Autodesk Inventor part; units mm, degrees
ref_plane "YZ Plane" through (0, 0, 0) normal (1, 0, 0) x (0, 1, 0)
ref_plane "XZ Plane" through (0, 0, 0) normal (0, 1, 0) x (-1, 0, 0)
ref_plane "XY Plane" through (0, 0, 0) normal (0, 0, 1) x (1, 0, 0)
sketch "Sketch1" plane through (0, 0, 0) normal (0, 1, 0) x (-1, 0, 0)
  line L0 (0, 0) -> (-12.7, 0)
  line L1 (-12.7, 0) -> (-12.7, -19.05)
  line L2 (-12.7, -19.05) -> (0, -19.05)
  line L3 (0, -19.05) -> (0, 0)
  line L4 (-12.7, -9.525) -> (0, -9.525)
  circle A0 centre (-6.35, -9.525) radius 3.175 construction
  dimension "d0" = 12.7
  dimension "d1" = 19.05
  dimension "d2" = 6.35
extrude "Extrusion1" add sketch "Sketch1" against normal blind 12.7
hole "Hole1" at (6.35, 0, -9.525) direction (0, -1, 0) diameter 5.1054 end through all counterbore diameter 9.525 counterbore depth 4.826
chamfer "Chamfer1" distance 0.4 angle 45 12 edges at (6.35, 0, -19.05) (12.7, 0, -9.525) (0, 0, -9.525) (6.35, 0, 0) (12.7, -6.35, 0) (12.7, -6.35, -19.05) (12.7, -12.7, -9.525) (6.35, -12.7, 0) (0, -6.35, 0) (0, -6.35, -19.05) (0, -12.7, -9.525) (6.35, -12.7, -19.05)
chamfer "Chamfer2" distance 0.2 angle 45 4 edges at (6.35, 0, -14.2875) (6.35, -12.7, -12.0777) (6.35, -4.826, -14.2875) (6.35, -4.826, -12.0777)
properties part number "Fixture Stop" material "ABS Plastic"
Geometry check sheet. Reference: the model listing, model coordinates, mm. A direction names the side the tool comes from. Give positions to 0.01 mm unless a question says otherwise; leave off trailing zeros. Write each loop counter-clockwise with the first axis right and the second up, starting at its lowest first coordinate (ties: lowest second). Pieces come first, ordered by that corner, then holes.
1) Release check for a two-part mould opening along Z. For faces 3 (the face through (12.7, -6, -9)), 4 (the face through (6, -6, -19.05)), 5 (the face through (5.58, -8.82, -7.09)), 6 (the face through (4.919, -2.444, -4.982)) record: released by +Z, released by -Z, zero draft, split by the parting line, or undercut.
Values follow:
face 3: zero draft
face 4: released by -Z
face 5: undercut
face 6: undercut
2) Thickness scan on line 1 (Z direction, x = 6.35, y = -3.05); line 2 (Z direction, x = 6.5, y = -5.75); line 3 (X direction, y = -3.25, z = -10.25). Record the ranges inside material, lowest first.
Values follow:
line 1: z = -19.05 to -14.29, -4.76 to 0
line 2: z = -19.05 to -12.07, -6.98 to 0
line 3: x = 0 to 1.64, 11.06 to 12.7
3) Cross-section at B-B (y = -5.25). Record the boundary of the cut face in (x, z) (3 decimals), plus the area to 3 significant figures.
Values follow:
outline: (0, -18.65) - (0.4, -19.05) - (12.3, -19.05) - (12.7, -18.65) - (12.7, -0.4) - (12.3, 0) - (0.4, 0) - (0, -0.4) - close; hole circle Ø5.105 at (6.35, -9.525)
area: 221 mm2
4) Cross-section at A-A (x = 6.35). Record the boundary of the cut face in (y, z).
Values follow:
outline: (-12.7, -18.65) - (-12.3, -19.05) - (-0.4, -19.05) - (0, -18.65) - (0, -14.49) - (-0.2, -14.29) - (-4.63, -14.29) - (-4.83, -14.09) - (-4.83, -12.28) - (-5.03, -12.08) - (-12.5, -12.08) - (-12.7, -12.28) - close; (-12.7, -6.77) - (-12.5, -6.97) - (-5.03, -6.97) - (-4.83, -6.77) - (-4.83, -4.96) - (-4.63, -4.76) - (-0.2, -4.76) - (0, -4.56) - (0, -0.4) - (-0.4, 0) - (-12.3, 0) - (-12.7, -0.4) - close
5) Set-up check for faces 1 (the face through (0, -6, -10)), 2 (the face through (6.3, -4.826, -6.5)): record each of +Z, -Z, +X, -X, +Y, -Y from which the full face is reachable in a straight line by a thin tool's end or side.
Values follow:
face 1: +Z, -Z, -X, +Y, -Y
face 2: +Y
